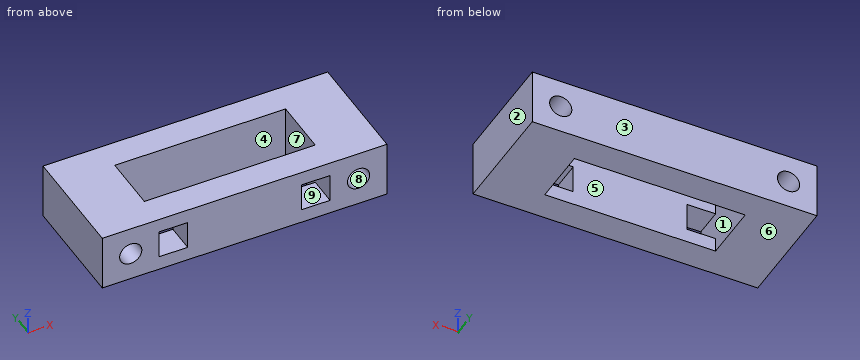
Solid Edge part; units mm, degrees
sketch "Sketch1" plane through (0, 0, 0) normal (0, -1, 0) x (1, 0, 0)
  line L0 (-25, -5) -> (25, -5)
  line L1 (25, -5) -> (25, 5)
  line L2 (25, 5) -> (-25, 5)
  line L3 (-25, 5) -> (-25, -5)
  dimension "D1" = 25
extrude "Protrusion1" add sketch "Sketch1" against normal blind 20
sketch "Sketch2" plane through (0, 0, 0) normal (0, -1, 0) x (1, 0, 0)
  circle A0 centre (-20, 0) radius 1.948
  circle A1 centre (20, 0) radius 1.948
extrude "Cutout1" cut sketch "Sketch2" against normal through all
sketch "Sketch3" plane through (0, 0, 0) normal (0, -1, 0) x (1, 0, 0)
  line L0 (-15, 5) -> (15, 5)
  line L1 (15, 5) -> (15, -5)
  line L2 (15, -5) -> (-15, -5)
  line L3 (-15, -5) -> (-15, 5)
extrude "Extrusionsausschnitt_3" cut sketch "Sketch3" against normal blind 15
sketch "Sketch4" plane through (-15, 7.5, 0) normal (1, 0, 0) x (0, 1, 0)
  line L0 (-7.5, 5) -> (-2.5, 5)
  line L1 (-2.5, 5) -> (-2.5, -5)
  line L2 (-2.5, -5) -> (-7.5, -5)
  line L3 (-7.5, -5) -> (-7.5, 5)
  dimension "D1" = 7.5
extrude "Extrusionsausprägung_2" add sketch "Sketch4" along normal blind 30
sketch "Sketch5" plane through (0, 0, 0) normal (0, -1, 0) x (1, 0, 0)
  line L0 (-15, -2.5) -> (-10, -2.5)
  line L1 (-10, -2.5) -> (-10, 2.5)
  line L2 (-10, 2.5) -> (-15, 2.5)
  line L3 (-15, 2.5) -> (-15, -2.5)
  line L4 (15, -2.5) -> (10, -2.5)
  line L5 (10, -2.5) -> (10, 2.5)
  line L6 (10, 2.5) -> (15, 2.5)
  line L7 (15, 2.5) -> (15, -2.5)
  dimension "D1" = 10
extrude "Cutout2" cut sketch "Sketch5" against normal up to next
properties material "Nylon, allgemein"
Work out the finished part from the listing and answer in its coordinate system (mm). Face numbers are marked on the shaded views. A direction names the side the tool comes from. Give positions to 0.01 mm unless a question says otherwise; leave off trailing zeros. Order: outer loops, then holes, each group sorted by start corner. A loop starts at its lowest first (then second) coordinate and runs counter-clockwise, first axis right, second up. Notation, with made-up numbers: (74, -1.5) - (95, -1.5) arc R30 cw to (95, 30.5) - close; hole circle Ø4 at (-13, -19). An arc over 180 degrees is marked (long way). Answer as CSV lines item,"result". Start each with the question number.
Q1. The part is cut by section C-C (x = -20). Write down the section's boundary in (y, z).
Q2. Find the intervals of material crossed by L1, parallel to Z at x = 20, y = 6.25; L2, parallel to X at y = 12.75, z = -4.5; L3, parallel to X at y = 11.5, z = 0.5, in increasing order. Write a range as [from, to].
Q3. The part is cut by section B-B (y = 11.75). Write down the section's boundary in (x, z), then the cut area to 3 significant figures.
Q4. The part is cut by section D-D (z = -3.75). Write down the section's boundary in (x, y).
Q5. For the marked faces 5, 6, 7, 8 and 9, determine the directions among +Z, -Z, +X, -X, +Y, -Y from which every point of the face is accessible in a straight line to the end or side of a thin tool.
Q6. The part is cut by section A-A (z = 0). Write down the section's boundary in (x, y).
Q7. Given pin 1 Ø3 at (x, z) = (20, 0) entering from -Y; pin 2 Ø6 at (x, z) = (-18.5, -3) entering from -Y, each flat-ended and moving along its own axis, determine where each tip first touches the part or whether it passes through.
Q8. The mould has two halves that part along X. Classify the marked faces 1, 2, 3 and 4: +X half, -X half, draft (parallel to the pull), parting line (faces both ways), or undercut.
Check result:
1,outline,"(0, -5) - (20, -5) - (20, -1.95) - (0, -1.95) - close; (0, 1.95) - (20, 1.95) - (20, 5) - (0, 5) - close"
2,L1,"z = [-5, -1.95], [1.95, 5]"
2,L2,"x = [-25, -15], [15, 25]"
2,L3,"x = [-25, -21.88], [-18.12, -15], [15, 18.12], [21.88, 25]"
3,outline,"(-25, -5) - (-15, -5) - (-15, 5) - (-25, 5) - close; (15, -5) - (25, -5) - (25, 5) - (15, 5) - close; hole circle Ø3.9 at (-20, 0); hole circle Ø3.9 at (20, 0)"
3,area,"176 mm²"
4,outline,"(-25, 0) - (25, 0) - (25, 20) - (-25, 20) - close; hole (-15, 5) - (15, 5) - (15, 15) - (-15, 15) - close"
5,face 5,"+Z, -Z"
5,face 6,"-Z, +X, -X, +Y, -Y"
5,face 7,"none"
5,face 8,"+Y, -Y"
5,face 9,"-Y"
6,outline,"(-25, 0) - (-21.95, 0) - (-21.95, 20) - (-25, 20) - close; (-18.05, 0) - (-15, 0) - (-15, 15) - (15, 15) - (15, 0) - (18.05, 0) - (18.05, 20) - (-18.05, 20) - close; (-10, 0) - (10, 0) - (10, 5) - (-10, 5) - close; (21.95, 0) - (25, 0) - (25, 20) - (21.95, 20) - close"
7,pin 1,"passes through"
7,pin 2,"stops at y = 0"
8,face 1,"undercut"
8,face 2,"+X half"
8,face 3,"draft"
8,face 4,"undercut"
